from build123d import *

# Parameters (mm, degrees)
RADIAL_BOLTS_COUNT = 6


with BuildPart() as part:
    # Sketch1 → base_revolve (revolve)
    with BuildSketch(Plane.XY, mode=Mode.PRIVATE) as base_revolve_sk:
        Polygon((0, 0), (2.54, 0), (16.129, -19.407103264), (16.129, -21.947103264), (7.566605976, -62.23), (5.026605976, -62.23), (12.855064142, -25.4), (0, -25.4), (0, -6.35), (1.27, -6.35), (1.27, -5.08), (0, -5.08), (0, -3.81), (1.27, -3.81), (1.27, -2.54), (0, -2.54), align=None)
    revolve(base_revolve_sk.sketch.rotate(Axis((20.32, 0, 0), (0, -1, 0)), 270), axis=Axis((20.32, 0, 0), (0, -1, 0)))

    # Sketch3 → 1/4 (0.25) Diameter Hole1 (revolve, cut)
    with BuildSketch(Plane(origin=(40.64, -19.05, 0), x_dir=(0, 0, -1), z_dir=(0, 1, 0))):
        Polygon((0, 0), (0, 8.89), (3.175, 6.982267535), (3.175, 0), align=None)
    f_1_4_0_25_diameter_hole1 = revolve(axis=Axis((46.99, -19.05, 0), (-1, 0, 0)), mode=Mode.SUBTRACT)

    # radial_bolts: 1/4 (0.25) Diameter Hole1 ×6 about axis
    radial_bolts_axis = Axis((20.32, 0, 0), (0, 1, 0))
    for i in range(1, RADIAL_BOLTS_COUNT):
        add(f_1_4_0_25_diameter_hole1.rotate(radial_bolts_axis, i * 360 / RADIAL_BOLTS_COUNT), mode=Mode.SUBTRACT)


solid = part.part
The model under review builds one solid part; all positions refer to its coordinate system, in mm. A direction names the side the tool comes from. Coordinates: 2 decimals unless noted, no trailing zeros. Loops run counter-clockwise (first coordinate to the right, second up) from the corner with the lowest first, then second, coordinate; pieces in that order, holes last. Notation, with made-up numbers: M 41.25,-1 L 96.25,-1 A22 cw 96.25,35 Z; hole C 26,7 d9. An arc over 180 degrees is marked long. Put each result on its own line as item: value. Start each with the question number.
Q1. For faces 4 (the flat face through (2, -5.08, -6)), 5 (the conical face through (8.559, -18.512, -0.12)), 6 (the cylindrical face through (37.2, -15.95, 0.69)), list the 3-axis set-ups (+Z, -Z, +X, -X, +Y, -Y) from which the entire face can be reached by the end or side of a thin tool; tool diameter is ignored.
Q2. Add section C-C (y = -8.5). Write out the cut boundary in (x, z), and give its area (3 significant figures).
Q3. Add section B-B (y = -55). Write out the cut boundary in (x, z).
Q4. Clearance check with flat-ended pins moving along their axes: pin 1 (8 mm diameter, centred on x = 30.5, y = -33.5, fed in from +Z); pin 2 (4 mm diameter, centred on x = 13, z = -6.5, fed in from +Y); pin 3 (6 mm diameter, centred on x = 24.5, y = -18.5, fed in from +Z); pin 4 (6.5 mm diameter, centred on x = 20.32, z = 0, fed in from -Y). State where each tip first meets the part, or that it passes through.
Q5. Wall thickness on line 1 (Z direction, x = 4.25, y = -19.05) (3 decimals); line 2 (X direction, y = -7.5, z = -8.5); line 3 (X direction, y = -20.7, z = 0): over which ranges is each line inside the solid? List them lowest first.
Q6. The part is to be moulded in two halves that separate along Z. For faces 1 (the flat face through (2, -3.81, 6)), 2 (the conical face through (17.96, -14.15, 7.51)), 3 (the cylindrical face through (0.173, -15.742, -2.645)), say which applies: +Z half, -Z half, draft (parallel to the pull), parting line (faces both ways), or undercut.
Answers:
1. face 4: none
1. face 5: -X
1. face 6: +X
2. outline: C 20.32,0 d40.64; hole C 20.32,0 d23.66
2. area: 858 mm^2
3. outline: C 20.32,0 d27.51; hole C 20.32,0 d22.43
4. pin 1: stops at z = 6.97
4. pin 2: stops at y = -8.56
4. pin 3: stops at z = 20.29
4. pin 4: passes through
5. line 1: z = -12.436 to -3.175, 3.175 to 12.436
5. line 2: x = 1.86 to 11.12, 29.52 to 38.78
5. line 3: x = 7.9 to 16.13, 24.51 to 32.74
6. face 1: draft
6. face 2: undercut
6. face 3: parting line
